Build history of the part. All positions in model axes, mm. A direction names the side the tool comes from. Give positions to 0.01 mm unless a question says otherwise; leave off trailing zeros. Write each loop counter-clockwise with the first axis right and the second up, starting at its lowest first coordinate (ties: lowest second). Pieces come first, ordered by that corner, then holes. Notation, with made-up numbers: (3, 31.5) -> (19, 31.5) arc R24 cw to (19, 41.5) -> close; hole circle Ø1 at (2.25, 35.5). An arc over 180 degrees is marked (long way). Write item = value, one per line. Start each with the question number.
Q1. Saw through at B-B, the plane x = -45. List the corners of the cut face in (y, z).
Q2. Wall check: line 1 (Z direction, x = -55, y = 0); line 2 (Z direction, x = -17, y = 5.5). Give the ranges that are in metal, low to high.
Q3. Saw through at D-D, the plane x = 18. List the corners of the cut face in (y, z).
Q4. Mould opens along Z. For faces 5 (the face through (17, -11, 7)), 6 (the face through (4, 0, 11.5)), 7 (the face through (-13, 0, 0)), 8 (the face through (-56.695, 26.846, 5.961)) say: pulls with the +Z half, pulls with the -Z half, needs draft (parallel to the pull), parting line crosses it, or undercut.
Q5. Saw through at A-A, the plane z = 0. List the corners of the cut face in (x, y), then the cut area to 3 significant figures.
Q6. Saw through at C-C, the plane y = 0. List the corners of the cut face in (x, z), then the cut area to 3 significant figures.
Q7. Tool access for faces 1 (the face through (34.116, 0.154, -0.524)), 2 (the face through (3, 0, -11.5)), 3 (the face through (-62.3, 12.864, -6.691)), 4 (the face through (17, 11, 7)): list every direction of +Z, -Z, +X, -X, +Y, -Y with a clear straight run to the whole face (end or side of a thin tool).
Q8. Drop flat-ended pins along their axis: P1, Ø16, axis at x = 19.5, z = 6.5, coming from the -Y side; P2, Ø5, axis at x = 15, z = -5.5, coming from the +Y side; P3, Ø1, axis at x = 18.5, y = -9.5, coming from the +Z side. Give the stop position or say it passes through.
from build123d import *

# Parameters (mm, degrees)
SKETCH2_R           = 6
BOSS_EXTRUDE1_DEPTH = 11


with BuildPart() as part:
    # Sketch1 → Revolve1 (revolve)
    with BuildSketch(Plane(origin=(0, 0, 0), x_dir=(1, 0, 0), z_dir=(0, 1, 0))):
        Polygon((0, 0), (-13, 0), (-13, 12.5), (-113, 12.5), (-113, 14.5), (-13, 14.5), (-13, 26.5), (-115, 26.5), (-115, 27.5), (0, 27.5), align=None)
    revolve(axis=Axis((0, 0, 0), (-1, 0, 0)))

    # Sketch2 → Boss-Extrude1 (add, symmetric)
    with BuildSketch(Plane(origin=(0, 0, 0), x_dir=(1, 0, 0), z_dir=(0, 1, 0))):
        with BuildLine():
            Line((0, 11.5), (7, 11.5))
            ThreePointArc((7, 11.5), (34.124297731, 0), (7, -11.5))
            Line((7, -11.5), (0, -11.5))
            Line((0, -11.5), (0, 11.5))
        make_face()
        with Locations((18.124297731, 0)):
            Circle(SKETCH2_R, mode=Mode.SUBTRACT)
    extrude(amount=BOSS_EXTRUDE1_DEPTH, both=True)


solid = part.part
Report:
q1.outline = circle Ø55 at (0, 0); circle Ø29 at (0, 0); hole circle Ø53 at (0, 0); hole circle Ø25 at (0, 0)
q2.line_1 = -27.5 to -26.5, -14.5 to -12.5, 12.5 to 14.5, 26.5 to 27.5
q2.line_2 = -26.94 to -25.92, -13.42 to -11.22, 11.22 to 13.42, 25.92 to 26.94
q3.outline = (-11, -16) -> (11, -16) -> (11, -6) -> (-11, -6) -> close; (-11, 6) -> (11, 6) -> (11, 16) -> (-11, 16) -> close
q4.face_5 = needs draft
q4.face_6 = pulls with the +Z half
q4.face_7 = undercut
q4.face_8 = parting line crosses it
q5.outline = (-115, -27.5) -> (0, -27.5) -> (0, -11) -> (12.12, -11) -> (12.12, 11) -> (0, 11) -> (0, 27.5) -> (-115, 27.5) -> (-115, 26.5) -> (-13, 26.5) -> (-13, 14.5) -> (-113, 14.5) -> (-113, 12.5) -> (-13, 12.5) -> (-13, -12.5) -> (-113, -12.5) -> (-113, -14.5) -> (-13, -14.5) -> (-13, -26.5) -> (-115, -26.5) -> close; (24.12, -11) -> (34.12, -11) -> (34.12, 11) -> (24.12, 11) -> close
q5.area = 1,810 mm2
q6.outline = (-115, -27.5) -> (0, -27.5) -> (0, -11.5) -> (7, -11.5) arc R16 ccw (long way) to (7, 11.5) -> (0, 11.5) -> (0, 27.5) -> (-115, 27.5) -> (-115, 26.5) -> (-13, 26.5) -> (-13, 14.5) -> (-113, 14.5) -> (-113, 12.5) -> (-13, 12.5) -> (-13, -12.5) -> (-113, -12.5) -> (-113, -14.5) -> (-13, -14.5) -> (-13, -26.5) -> (-115, -26.5) -> close; hole circle Ø12 at (18.12, 0)
q6.area = 2,090 mm2
q7.face_1 = +Y, -Y
q7.face_2 = -Z, +Y, -Y
q7.face_3 = -X
q7.face_4 = +Z, -Z, +X, +Y
q8.P1 = -11
q8.P2 = 11
q8.P3 = 16
